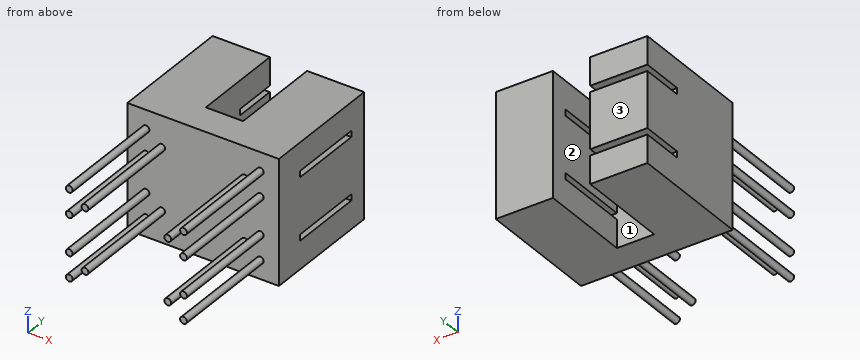
from build123d import *

# Parameters (mm, degrees)
SKETCH1_W               = 4.6
SKETCH1_H               = 5
BOSS_EXTRUDE1_DEPTH     = 7.5
BOSS_EXTRUDE1_2_DEPTH   = 7.5
SKETCH1_4_W             = 4.6
SKETCH1_4_H             = 5
SKETCH1_4_W_2           = 3
BOSS_EXTRUDE2_DEPTH     = 2.5
SKETCH2_W               = 0.5
SKETCH2_H               = 3.5
CUT_EXTRUDE1_DEPTH      = 11.966312051
SKETCH3_W               = 0.5
SKETCH3_H               = 6
CUT_EXTRUDE2_DEPTH      = 11.966312051
SKETCH5_R               = 0.275
BOSS_EXTRUDE3_DEPTH     = 9
MIRROR1_COPY_1_SKETCH_R = 0.275
MIRROR1_COPY_1_DEPTH    = 9


with BuildPart() as part:
    # Sketch1 → Boss-Extrude1 (new body)
    with BuildSketch(Plane(origin=(0, 0, 0), x_dir=(1, 0, 0), z_dir=(0, 1, 0))):
        with Locations((-3.8, 0)):
            Rectangle(SKETCH1_W, SKETCH1_H)
    boss_extrude1 = extrude(amount=BOSS_EXTRUDE1_DEPTH)



with BuildPart() as body_2:
    # Sketch1 → Boss-Extrude1 2 (new body)
    with BuildSketch(Plane(origin=(0, 0, 0), x_dir=(1, 0, 0), z_dir=(0, 1, 0))):
        with Locations((3.8, 0)):
            Rectangle(SKETCH1_W, SKETCH1_H)
    boss_extrude1_2 = extrude(amount=BOSS_EXTRUDE1_2_DEPTH)


with BuildPart() as part_1:
    add(part.part)

    add(body_2.part)  # Boss-Extrude2 merges body 2
    # Sketch1_4 → Boss-Extrude2 (add)
    with BuildSketch(Plane(origin=(0, 0, 0), x_dir=(1, 0, 0), z_dir=(0, 1, 0))):
        with Locations((-3.8, 0)):
            Rectangle(SKETCH1_4_W, SKETCH1_4_H)
        Rectangle(SKETCH1_4_W_2, SKETCH1_4_H)
        with Locations((3.8, 0)):
            Rectangle(SKETCH1_4_W, SKETCH1_4_H)
    boss_extrude2 = extrude(amount=-BOSS_EXTRUDE2_DEPTH)

    # Sketch2 → Cut-Extrude1 (cut, through all)
    with BuildSketch(Plane(origin=(-1.5, 0, 0), x_dir=(0, 0, -1), z_dir=(1, 0, 0))):
        with Locations((0, 5.75)):
            Rectangle(SKETCH2_W, SKETCH2_H)
    cut_extrude1 = extrude(amount=-CUT_EXTRUDE1_DEPTH, mode=Mode.SUBTRACT)

    # Sketch3 → Cut-Extrude2 (cut, through all)
    with BuildSketch(Plane.ZY.offset(-1.5)):
        with Locations((0, 3)):
            Rectangle(SKETCH3_W, SKETCH3_H)
    cut_extrude2 = extrude(amount=-CUT_EXTRUDE2_DEPTH, mode=Mode.SUBTRACT)

    # Sketch5 → Boss-Extrude3 (add)
    with BuildSketch(Plane(origin=(0, -2.5, 0), x_dir=(-1, 0, 0), z_dir=(0, -1, 0))):
        with Locations(Location((4.6, -1, 0), (0, 0, 270))):
            Circle(SKETCH5_R)
        with Locations(Location((4.6, 1, 0), (0, 0, 270))):
            Circle(SKETCH5_R)
        with Locations(Location((3.33, 0, 0), (0, 0, 270))):
            Circle(SKETCH5_R)
    boss_extrude3 = extrude(amount=BOSS_EXTRUDE3_DEPTH)

    # Mirror2: Boss-Extrude3 across plane
    add(boss_extrude3.mirror(Plane(origin=(0, 0, 0), x_dir=(0, 0, 1), z_dir=(1, 0, 0))))

    # Mirror1: Boss-Extrude1, Boss-Extrude1 2, Boss-Extrude2, Cut-Extrude1, Cut-Extrude2, Boss-Extrude3 across plane
    add(boss_extrude1.mirror(Plane(origin=(0, 7.5, -2.5), x_dir=(1, 0, 0), z_dir=(0, 0, 1))))
    add(boss_extrude1_2.mirror(Plane(origin=(0, 7.5, -2.5), x_dir=(1, 0, 0), z_dir=(0, 0, 1))))
    add(boss_extrude2.mirror(Plane(origin=(0, 7.5, -2.5), x_dir=(1, 0, 0), z_dir=(0, 0, 1))))
    add(cut_extrude1.mirror(Plane(origin=(0, 7.5, -2.5), x_dir=(1, 0, 0), z_dir=(0, 0, 1))), mode=Mode.SUBTRACT)
    add(cut_extrude2.mirror(Plane(origin=(0, 7.5, -2.5), x_dir=(1, 0, 0), z_dir=(0, 0, 1))), mode=Mode.SUBTRACT)
    add(boss_extrude3.mirror(Plane(origin=(0, 7.5, -2.5), x_dir=(1, 0, 0), z_dir=(0, 0, 1))))

    # Mirror1 copy 1 sketch → Mirror1 copy 1 (add)
    with BuildSketch(Plane(origin=(0, -2.5, -5), x_dir=(1, 0, 0), z_dir=(0, -1, 0))):
        with Locations(Location((4.6, -1, 0), (0, 0, 270))):
            Circle(MIRROR1_COPY_1_SKETCH_R)
        with Locations(Location((4.6, 1, 0), (0, 0, 270))):
            Circle(MIRROR1_COPY_1_SKETCH_R)
        with Locations(Location((3.33, 0, 0), (0, 0, 270))):
            Circle(MIRROR1_COPY_1_SKETCH_R)
    extrude(amount=MIRROR1_COPY_1_DEPTH)


solid = part_1.part
Verification items for the finished model (mm, model axes). Face numbers are marked on the shaded views. A direction names the side the tool comes from. Give positions to 0.01 mm unless a question says otherwise; leave off trailing zeros. Write each loop counter-clockwise with the first axis right and the second up, starting at its lowest first coordinate (ties: lowest second). Pieces come first, ordered by that corner, then holes.
(1) Access from +Z, -Z, +X, -X, +Y, -Y to the whole of each face (thin tool, end or side, straight path). Record for the marked faces 1, 2 and 3.
(2) Cross-section at C-C (y = 3.25). Enter the section's corners in (x, z).
(3) Cross-section at D-D (x = -4.6). Enter the section's corners in (y, z) (3 decimals).
(4) Material ranges on line 1 (X direction, y = 4, z = -4.25); line 2 (X direction, y = -4, z = -5) (3 decimals); line 3 (Y direction, x = -0.75, z = 2), recorded low to high.
(5) Cross-section at A-A (z = -5). Enter the section's corners in (x, y) (3 decimals), plus the area to 3 significant figures.
(6) Gauge pin test, flat ends, axial feed: pin 1 (2 mm diameter, centred on x = -3, y = -6, fed in from +Z) (3 decimals); pin 2 (1 mm diameter, centred on x = -1, z = -6, fed in from -Y); pin 3 (1 mm diameter, centred on x = 0.5, z = -5.5, fed in from +Y). Record the tip position at first contact, or that the pin passes through.
(7) Cross-section at B-B (y = -5.25). State how many separate pieces and enclosed holes the cut face has, plus the area to 3 significant figures.
Worked out:
1. face 1: none
1. face 2: +Z, -Z, +Y
1. face 3: +Z, -Z, +X, -X, +Y
2. outline: (-6.1, -7.5) - (-1.5, -7.5) - (-1.5, 2.5) - (-6.1, 2.5) - close; (1.5, -7.5) - (6.1, -7.5) - (6.1, -5.25) - (1.5, -5.25) - close; (1.5, -4.75) - (6.1, -4.75) - (6.1, -0.25) - (1.5, -0.25) - close; (1.5, 0.25) - (6.1, 0.25) - (6.1, 2.5) - (1.5, 2.5) - close
3. outline: (-11.5, -6.275) - (-2.5, -6.275) - (-2.5, -7.5) - (7.5, -7.5) - (7.5, -5.25) - (4, -5.25) - (4, -4.75) - (7.5, -4.75) - (7.5, -0.25) - (4, -0.25) - (4, 0.25) - (7.5, 0.25) - (7.5, 2.5) - (-2.5, 2.5) - (-2.5, 1.275) - (-11.5, 1.275) - (-11.5, 0.725) - (-2.5, 0.725) - (-2.5, -0.725) - (-11.5, -0.725) - (-11.5, -1.275) - (-2.5, -1.275) - (-2.5, -3.725) - (-11.5, -3.725) - (-11.5, -4.275) - (-2.5, -4.275) - (-2.5, -5.725) - (-11.5, -5.725) - close
4. line 1: x = -6.1 to -1.5, 1.5 to 6.1
4. line 2: x = -3.605 to -3.055, 3.055 to 3.605
4. line 3: y = -2.5 to 0
5. outline: (-6.1, -2.5) - (-3.605, -2.5) - (-3.605, -11.5) - (-3.055, -11.5) - (-3.055, -2.5) - (3.055, -2.5) - (3.055, -11.5) - (3.605, -11.5) - (3.605, -2.5) - (6.1, -2.5) - (6.1, 0) - (-1.5, 0) - (-1.5, 4) - (-6.1, 4) - close; (1.5, 6) - (6.1, 6) - (6.1, 7.5) - (1.5, 7.5) - close
5. area: 65.7 mm2
6. pin 1: stops at z = 0.275
6. pin 2: stops at y = -2.5
6. pin 3: stops at y = 0
7. separate pieces: 12
7. enclosed holes: 0
7. area: 2.85 mm2
